Here's how the part is built. I have some questions about the finished solid (model axes, mm). A direction names the side the tool comes from. Round coordinates to 2 decimals unless told otherwise and drop trailing zeros. Write each loop counter-clockwise with the first axis right and the second up, starting at its lowest first coordinate (ties: lowest second). Pieces come first, ordered by that corner, then holes. Notation, with made-up numbers: (-11, 43) -> (45, 43) arc R25 cw to (45, 58) -> close; hole circle Ø3 at (46.25, 18.5). An arc over 180 degrees is marked (long way). Answer as CSV lines item,"result".
Autodesk Inventor part; units mm, degrees
ref_plane "Work Plane1" through (17.5119, 0, 0) normal (0, 0, 1) x (-1, 0, 0)
ref_plane "YZ Plane" through (0, 0, 0) normal (1, 0, 0) x (0, 1, 0)
ref_plane "XZ Plane" through (0, 0, 0) normal (0, 1, 0) x (-1, 0, 0)
sketch "Sketch1" plane through (0, 0, 0) normal (1, 0, 0) x (0, 1, 0)
  line L0 (2.8868, -5) -> (-2.8868, -5)
  line L1 (-2.8868, -5) -> (-5.7735, 0)
  line L2 (-5.7735, 0) -> (-2.8868, 5)
  line L3 (-2.8868, 5) -> (2.8868, 5)
  line L4 (2.8868, 5) -> (5.7735, 0)
  line L5 (5.7735, 0) -> (2.8868, -5)
  point P0 (0, 0)
  point P1 (0, 0)
  dimension "d0" = 11.547
extrude "Body" add sketch "Sketch1" along normal blind 5.4
sketch "Sketch2" plane through (5.4, 0, 0) normal (1, 0, 0) x (0, 0, -1)
  circle A0 centre (0, 0) radius 4.44
  dimension "d7" = 8.88
extrude "Ring" add sketch "Sketch2" along normal blind 3.1
sketch "Sketch3" plane through (0, 0, 0) normal (0, 0, 1) x (1, 0, 0)
  line L0 (0, 2.8868) -> (0, 5.7735)
  line L1 (0, 5.7735) -> (5.4, 5.7735)
  line L2 (5.4, 2.8868) -> (5.4, 5.7735)
  line L3 (-1.08, 0) -> (6.48, 0)
  line L4 (0, 4.44) -> (0.7699, 5.7735)
  line L5 (4.6301, 5.7735) -> (5.4, 4.44)
  dimension "d3" = 30
  dimension "d4" = 30
  dimension "d5" = 8.88
  dimension "d6" = 8.88
revolve "Chamfer1" cut sketch "Sketch3" angle 360 about axis through (-10, 0, 0) along (1, 0, 0)
sketch "Sketch4" plane through (0, 0, 0) normal (-1, 0, 0) x (0, 0, 1)
  line L0 (0, -8.0829) -> (0, 8.0829)
  line L1 (-7, 0) -> (7, 0)
  point P0 (0, 0)
hole "Thread" at (0, 0, 0) direction (1, 0, 0) diameter 4.917 end through all
chamfer "Chamfer2" distance 0.5413 angle 30 1 edges at (0, 0, -2.4585) measured on face at (0, 3.7305, -0.453)
chamfer "Chamfer3" distance 0.5413 angle 30 1 edges at (8.5, 0, -2.4585) measured on face at (8.5, -0.5503, -3.7127)
ref_plane "Work Plane1" through (17.5119, 0, 0) normal (0, 0, 1) x (-1, 0, 0)
equation "\"d0\" = 1.1547 * SW"
equation "\"d1\" = KOH1"
equation "\"d7\" = SD2"
equation "\"d8\" = KOH - KOH1"
equation "\"d3\" = ANG1"
equation "\"d4\" = ANG2"
equation "\"d5\" = SW0"
equation "\"d6\" = SW01"
equation "\"d10\" = -0.5 * GD1 + 0.5 * NND"
equation "\"d46\" = -0.5 * GD1 + 0.5 * NND"
equation "\"d12\" = -0.5 * GD1 + 0.5 * NND"
equation "\"d47\" = -0.5 * GD1 + 0.5 * NND"
equation "\"ANG1\" = 30deg"
equation "\"ANG2\" = 30deg"
equation "\"NND\" = 6"
equation "\"KOH1\" = 5.4"
equation "\"KOH\" = 8.5"
equation "\"SW0\" = 8.88"
equation "\"SW01\" = SW0"
equation "\"SD2\" = SW0"
equation "\"GUL\" = 0.541266 * PTC"
equation "\"THREADDIA\" = 6"
equation "\"TOA\" = 30deg"
equation "\"PTC\" = 1"
equation "\"GAL\" = 0.541266 * PTC"
equation "\"E0\" = 1.155 * SW"
properties part number "ISO 7041 - M6" material "Steel"
Item 1: Suppose I cut it at A-A, the plane y = 0. List the corners of the cut face in (x, z) for me.
Results found:
outline,"(0, -4.44) -> (0.32, -5) -> (5.08, -5) -> (5.4, -4.44) -> (8.5, -4.44) -> (8.5, -3) -> (8.19, -2.46) -> (0.31, -2.46) -> (0, -3) -> close; (0, 3) -> (0.31, 2.46) -> (8.19, 2.46) -> (8.5, 3) -> (8.5, 4.44) -> (5.4, 4.44) -> (5.08, 5) -> (0.32, 5) -> (0, 4.44) -> close"
Item 2: Suppose I cut it at B-B, the plane x = 6.75. List the corners of the cut face in (y, z) for me, then the cut area to 3 significant figures.
Results found:
outline,"circle Ø8.88 at (0, 0); hole circle Ø4.92 at (0, 0)"
area,"42.9 mm²"
Item 3: For faces 1 (the cylindrical face through (6.928, 4.334, 0.963)), 2 (the flat face through (8.5, -3, -1)), which set-ups out of +Z, -Z, +X, -X, +Y, -Y let a thin tool reach every point of the face, with its end or its side?
Results found:
face 1,"+X"
face 2,"+Z, -Z, +X, +Y, -Y"
Item 4: If we mould it in two halves opening along Z, with no side actions, what happens to faces 3 (the flat face through (2.667, 4.31, 2.535)), 4 (the flat face through (2.667, 4.35, -2.465)), 5 (the cylindrical face through (4.305, -0.738, 2.345))? For each: pulls with the +Z half, pulls with the -Z half, needs draft (parallel to the pull), parting line crosses it, or undercut.
Results found:
face 3,"pulls with the +Z half"
face 4,"pulls with the -Z half"
face 5,"undercut"
Item 5: I need wall thicknesses on L1, parallel to Y at x = 6.5, z = 0; L2, parallel to Z at x = 2, y = 0. Which ranges of each line are inside material? Lowest first, please.
Results found:
L1,"y = -4.44 to -2.46, 2.46 to 4.44"
L2,"z = -5 to -2.46, 2.46 to 5"
Item 6: Suppose I cut it at C-C, the plane x = 1. List the corners of the cut face in (y, z) for me, then the cut area to 3 significant figures.
Results found:
outline,"(-5.77, 0) -> (-2.89, -5) -> (2.89, -5) -> (5.77, 0) -> (2.89, 5) -> (-2.89, 5) -> close; hole circle Ø4.92 at (0, 0)"
area,"67.6 mm²"
Item 7: Will these pins go through, and if not, where does the flat tip stop? pin 1 (4 mm diameter, centred on x = 4.5, z = 3, fed in from -Y); pin 2 (1 mm diameter, centred on x = 5, z = -2, fed in from +Y); pin 3 (4.5 mm diameter, centred on y = 0, z = 0, fed in from -X).
Results found:
pin 1,"stops at y = -5.2"
pin 2,"stops at y = 4.91"
pin 3,"passes through"
